Part print with two shaded views. Sizes in mm from the minimum x, y, z corner. A direction names the side the tool comes from. Coordinates: 2 decimals unless noted, no trailing zeros. Loops run counter-clockwise (first coordinate to the right, second up) from the corner with the lowest first, then second, coordinate; pieces in that order, holes last. Notation, with made-up numbers: (5, -29.75) - (9, -29.75) arc R9 ccw to (9, -17.75) - close; hole circle Ø4 at (70.25, -34). An arc over 180 degrees is marked (long way). Answer as CSV lines item,"result".
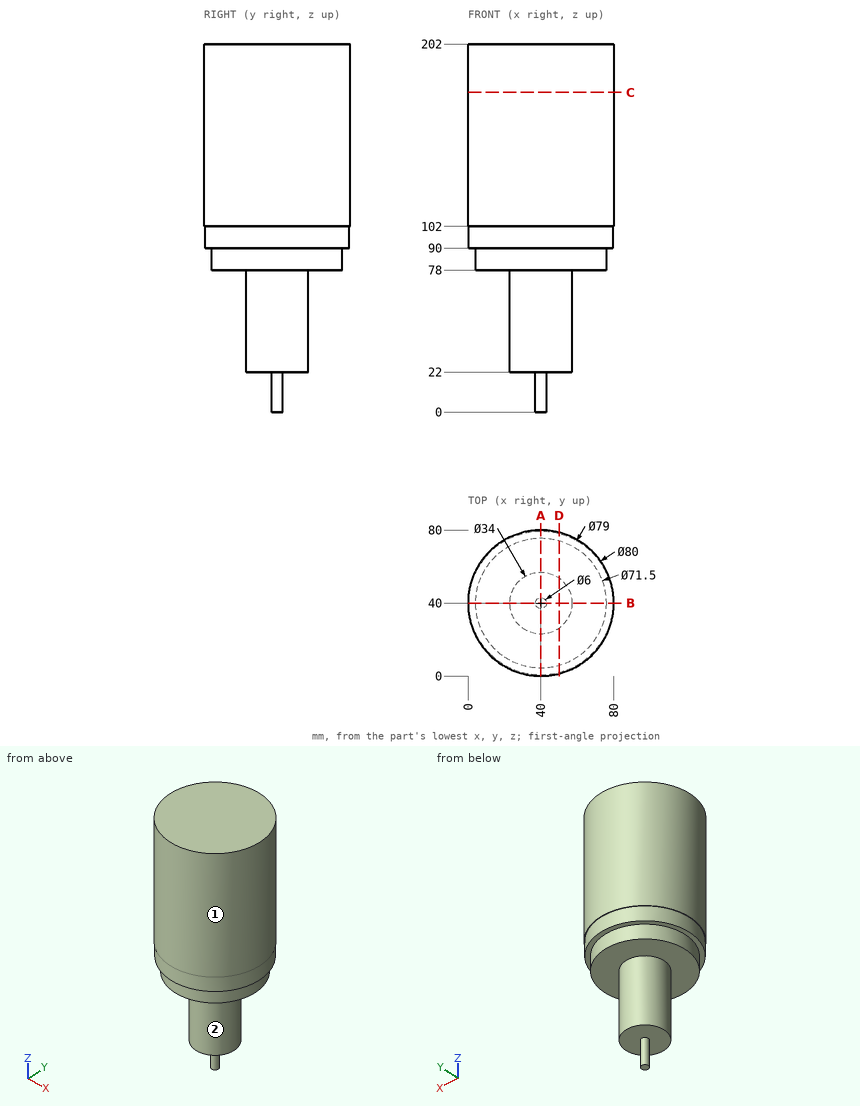
Q1. Saw through at C-C (z = 175.5). Give the cut face in (x, y), then the cut area to 3 significant figures.
Results:
outline,"circle Ø80 at (40, 40)"
area,"5,030 mm^2"
Q2. Wall check: L1, parallel to Z at x = 37.5, y = 69; L2, parallel to Z at x = 69.5, y = 60.5; L3, parallel to Y at x = 39, z = 133. Give the ranges that are in metal, low to high.
Results:
L1,"z = 78 to 202"
L2,"z = 90 to 202"
L3,"y = 0.01 to 79.99"
Q3. Saw through at D-D (x = 50). Give the cut face in (y, z), then the cut area to 3 significant figures.
Results:
outline,"(1.27, 102) - (1.79, 102) - (1.79, 90) - (5.68, 90) - (5.68, 78) - (26.25, 78) - (26.25, 22) - (53.75, 22) - (53.75, 78) - (74.32, 78) - (74.32, 90) - (78.21, 90) - (78.21, 102) - (78.73, 102) - (78.73, 202) - (1.27, 202) - close"
area,"11,000 mm^2"
Q4. Flat gauge pins, fed straight in: pin 1 (4 mm diameter, centred on x = 28.5, z = 113.5, fed in from +Y); pin 2 (12 mm diameter, centred on x = 70, z = 103.5, fed in from +Y); pin 3 (10 mm diameter, centred on y = 37, z = 48, fed in from +X). Where does each tip first touch, or does it go through?
Results:
pin 1,"stops at y = 78.86"
pin 2,"stops at y = 72"
pin 3,"stops at x = 57"
Q5. Which spindle directions (+Z, -Z, +X, -X, +Y, -Y) get a long thin tool onto all of the face, cutting with end or side? Do the marked faces 1 and 2. Say none if no direction does.
Results:
face 1,"+Z, -Z"
face 2,"-Z"
Q6. Saw through at A-A (x = 40). Give the cut face in (y, z), then the cut area to 3 significant figures.
Results:
outline,"(0, 102) - (0.5, 102) - (0.5, 90) - (4.25, 90) - (4.25, 78) - (23, 78) - (23, 22) - (37, 22) - (37, 0) - (43, 0) - (43, 22) - (57, 22) - (57, 78) - (75.75, 78) - (75.75, 90) - (79.5, 90) - (79.5, 102) - (80, 102) - (80, 202) - (0, 202) - close"
area,"11,800 mm^2"
